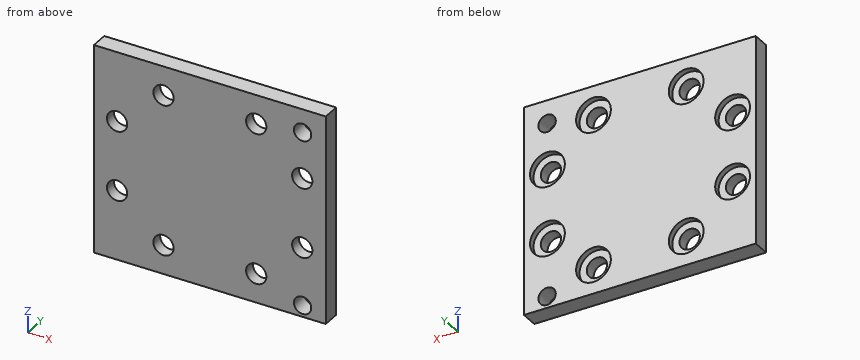
Autodesk Inventor part; units mm, degrees
ref_plane "YZ Plane" through (0, 0, 0) normal (1, 0, 0) x (0, 1, 0)
ref_plane "XZ Plane" through (0, 0, 0) normal (0, 1, 0) x (-1, 0, 0)
ref_plane "XY Plane" through (0, 0, 0) normal (0, 0, 1) x (1, 0, 0)
sketch "Sketch1" plane through (0, 0, 0) normal (0, 1, 0) x (-1, 0, 0)
  line L0 (0, 0) -> (-40, 0)
  line L1 (-40, 0) -> (-40, -36)
  line L2 (-40, -36) -> (0, -36)
  line L3 (0, -36) -> (0, 0)
  line L4 (0, 0) -> (0, -5)
  circle A0 centre (-12, -5) radius 3
  circle A1 centre (-28, -5) radius 3
  line L5 (0, 0) -> (-4, 0)
  circle A2 centre (-4, -12) radius 3
  line L6 (-40, 0) -> (-36, 0)
  line L7 (-40, -4) -> (-40, 0)
  circle A3 centre (-36, -4) radius 1.5
  circle A4 centre (-4, -24) radius 3
  circle A5 centre (-12, -31) radius 3
  circle A6 centre (-28, -31) radius 3
  circle A7 centre (-36, -34) radius 1.5
  dimension "d0" = 40
  dimension "d1" = 36
  dimension "d11" = 6
  dimension "d13" = 0
  dimension "d14" = 0
  dimension "d15" = 5
  dimension "d16" = 4
  dimension "d17" = 4
  dimension "d18" = 12
  dimension "d19" = 4
  dimension "d20" = 24
  dimension "d21" = 12
  dimension "d22" = 5
  dimension "d23" = 12
  dimension "d24" = 31
  dimension "d25" = 28
  dimension "d26" = 5
  dimension "d27" = 28
  dimension "d29" = 36
  dimension "d30" = 36
  dimension "d31" = 4
  dimension "d32" = 36
  dimension "d34" = 4
  dimension "d88" = 30
  dimension "d89" = 3
extrude "Extrusion1" add sketch "Sketch1" along normal blind 3
sketch "Sketch2" plane through (0, 3, 0) normal (0, 1, 0) x (1, 0, 0)
  line L0 (39.9397, 0) -> (35.9397, 0)
  line L1 (0, 0) -> (40, 0)
  line L2 (35.9397, 0) -> (35.9397, 12)
  line L3 (35.9397, 12) -> (35.9397, 24)
  circle A0 centre (35.9397, 12) radius 3
  circle A1 centre (35.9397, 24) radius 3
  dimension "d4" = 4
  dimension "d5" = 12
  dimension "d6" = 12
  dimension "d7" = 6
  dimension "d8" = 6
  dimension "d35" = 0
  dimension "d36" = 35.9397
  dimension "d37" = 4.0603
  dimension "d38" = 35.9397
extrude "Extrusion2" cut sketch "Sketch2" against normal blind 3
sketch "Sketch5" plane through (0, 0, 0) normal (0, -1, 0) x (1, 0, 0)
  circle A0 centre (12, -5) radius 1.75
  circle A1 centre (12, -5) radius 3
  circle A2 centre (12, -5) radius 3
  circle A3 centre (28, -5) radius 1.75
  circle A4 centre (28, -5) radius 3
  circle A5 centre (28, -5) radius 3
  circle A6 centre (4, -12) radius 1.75
  circle A7 centre (4, -12) radius 3
  circle A8 centre (4, -12) radius 3
  circle A9 centre (35.9397, -12) radius 1.75
  circle A10 centre (35.9397, -12) radius 3
  circle A11 centre (35.9397, -24) radius 3
  circle A12 centre (28, -31) radius 3
  circle A13 centre (12, -31) radius 3
  circle A14 centre (4, -24) radius 3
  circle A15 centre (4, -12) radius 3
  circle A16 centre (28, -5) radius 3
  circle A17 centre (12, -5) radius 3
  circle A18 centre (36, -34) radius 1.5
  circle A19 centre (36, -4) radius 1.5
  line L0 (0, 0) -> (40, 0)
  line L1 (0, -36) -> (0, 0)
  line L2 (40, -36) -> (0, -36)
  line L3 (40, 0) -> (40, -36)
  circle A20 centre (35.9397, -12) radius 3
  circle A21 centre (35.9397, -24) radius 1.75
  circle A22 centre (35.9397, -24) radius 3
  circle A23 centre (28, -31) radius 1.75
  circle A24 centre (28, -31) radius 3
  circle A25 centre (12, -31) radius 1.75
  circle A26 centre (12, -31) radius 3
  circle A27 centre (4, -24) radius 1.75
  circle A28 centre (4, -24) radius 3
  circle A29 centre (4, -24) radius 3
  point P0 (-35.9397, 24)
  point P1 (-28, 31)
  point P2 (-28, 31)
  point P3 (-28, 31)
  dimension "d39" = 3.5
  dimension "d40" = 0
  dimension "d41" = 0
  dimension "d42" = 3.5
  dimension "d43" = 0
  dimension "d44" = 0
  dimension "d45" = 6
  dimension "d46" = 3.5
  dimension "d47" = 0
  dimension "d48" = 0
  dimension "d49" = 6
  dimension "d50" = 3.5
  dimension "d51" = 0
  dimension "d52" = 0
  dimension "d53" = 6
  dimension "d54" = 3.5
  dimension "d55" = 0
  dimension "d56" = 0
  dimension "d57" = 6
  dimension "d58" = 3.5
  dimension "d59" = 0
  dimension "d60" = 0
  dimension "d61" = 6
  dimension "d62" = 3.5
  dimension "d63" = 0
  dimension "d64" = 0
  dimension "d65" = 6
  dimension "d66" = 3.5
  dimension "d67" = 0
  dimension "d68" = 0
  dimension "d69" = 6
  dimension "d74" = 68
  dimension "d75" = 67
  dimension "d76" = 68
  dimension "d77" = 67
  dimension "d78" = 68
  dimension "d79" = 67
  dimension "d80" = 75.9397
  dimension "d81" = 60
extrude "Extrusion4" add sketch "Sketch5" against normal blind 2 contours A1 | A4 | A7 | A10 | A11 | A12 | A13 | A14
properties part number "reverse gear steam chest cover"
Work out the finished part from the listing and answer in its coordinate system (mm). Coordinates: 2 decimals unless noted, no trailing zeros. Loops run counter-clockwise (first coordinate to the right, second up) from the corner with the lowest first, then second, coordinate; pieces in that order, holes last. Notation, with made-up numbers: (76.25, 53.5) -> (133.25, 53.5) arc R21 cw to (133.25, 70.5) -> close; hole circle Ø2 at (80.5, 70.5). An arc over 180 degrees is marked (long way). Answer as CSV lines item,"result".
1) The part is cut by section D-D (z = -5). Give the vertices of the cut face in (x, y), and give its area (3 significant figures).
A:
outline,"(0, 0) -> (10.25, 0) -> (10.25, 2) -> (9, 2) -> (9, 3) -> (0, 3) -> close; (13.75, 0) -> (26.25, 0) -> (26.25, 2) -> (25, 2) -> (25, 3) -> (15, 3) -> (15, 2) -> (13.75, 2) -> close; (29.75, 0) -> (34.88, 0) -> (34.88, 3) -> (31, 3) -> (31, 2) -> (29.75, 2) -> close; (37.12, 0) -> (40, 0) -> (40, 3) -> (37.12, 3) -> close"
area,"87.3 mm²"
2) Straight lines are drawn through the part: probe 1 along Z at (x, y) = (12, 2.5); probe 2 along Z at (x, y) = (4, 2.6); probe 3 along X at (y, z) = (0.75, -24.5). For each, find the intervals that lie inside material, in ascending order.
A:
probe 1,"z = -36 to -34, -28 to -8, -2 to 0"
probe 2,"z = -36 to -27, -21 to -15, -9 to 0"
probe 3,"x = 0 to 2.32, 5.68 to 34.26, 37.62 to 40"
3) The part is cut by section B-B (y = 1.55). State how many separate pieces and enclosed holes the cut face has, and give its area (3 significant figures).
A:
separate pieces,"1"
enclosed holes,"10"
area,"1,350 mm²"
4) The part is cut by section C-C (x = 12). Give the vertices of the cut face in (y, z).
A:
outline,"(0, -36) -> (3, -36) -> (3, -34) -> (2, -34) -> (2, -32.75) -> (0, -32.75) -> close; (0, -29.25) -> (2, -29.25) -> (2, -28) -> (3, -28) -> (3, -8) -> (2, -8) -> (2, -6.75) -> (0, -6.75) -> close; (0, -3.25) -> (2, -3.25) -> (2, -2) -> (3, -2) -> (3, 0) -> (0, 0) -> close"
5) The part is cut by section A-A (z = -12). Give the vertices of the cut face in (x, y).
A:
outline,"(0, 0) -> (2.25, 0) -> (2.25, 2) -> (1, 2) -> (1, 3) -> (0, 3) -> close; (5.75, 0) -> (34.19, 0) -> (34.19, 2) -> (32.94, 2) -> (32.94, 3) -> (7, 3) -> (7, 2) -> (5.75, 2) -> close; (37.69, 0) -> (40, 0) -> (40, 3) -> (38.94, 3) -> (38.94, 2) -> (37.69, 2) -> close"
6) Flat-ended cylindrical pins translate along their axes: pin 1 (3 mm diameter, centred on x = 12, z = -5, fed in from -Y); pin 2 (5 mm diameter, centred on x = 28, z = -31, fed in from +Y). Find the tip coordinate at first contact, or state that the pin passes through.
A:
pin 1,"passes through"
pin 2,"stops at y = 2"
